Input: part model. Units: mm. Frame: model coordinates. Face numbers are marked on the shaded views. A direction names the side the tool comes from. Give positions to 0.01 mm unless a question says otherwise; leave off trailing zeros. Loops run counter-clockwise (first coordinate to the right, second up) from the corner with the lowest first, then second, coordinate; pieces in that order, holes last. Notation, with made-up numbers: (-31, -0.5) -> (11, -0.5) arc R21 cw to (11, 16.5) -> close; hole circle Ø9 at (-21.75, -36). An arc over 180 degrees is marked (long way). Answer as a JSON object with one key per item and string values.
```python
from build123d import *

# Parameters (mm, degrees)
SKETCH1_W   = 19.939
SKETCH1_H   = 40.2844
BODY_DEPTH  = 39.7002
SKETCH2_R   = 2.921
AXLE_DEPTH  = 5.6896
WINGS_START = 28.448
SKETCH3_W   = 19.939
SKETCH3_H   = 7.112
SKETCH3_R   = 2.159
WINGS_DEPTH = 3


with BuildPart() as part:
    # Sketch1 → Body (new body)
    with BuildSketch(Plane(origin=(0, 0, 0), x_dir=(1, 0, 0), z_dir=(0, 1, 0))):
        with Locations((0, -10.1422)):
            Rectangle(SKETCH1_W, SKETCH1_H)
    extrude(amount=BODY_DEPTH)

    # Sketch2 → Axle (add)
    with BuildSketch(Plane(origin=(0, 39.7002, 0), x_dir=(1, 0, 0), z_dir=(0, 1, 0))):
        Circle(SKETCH2_R)
    extrude(amount=AXLE_DEPTH)

    # Sketch3 → Wings (add)
    with BuildSketch(Plane(origin=(0, 0, 0), x_dir=(1, 0, 0), z_dir=(0, 1, 0)).offset(WINGS_START)):
        with Locations((0, 13.556)):
            Rectangle(SKETCH3_W, SKETCH3_H)
        with Locations((4.98475, 14.2672)):
            Circle(SKETCH3_R, mode=Mode.SUBTRACT)
        with Locations((-4.98475, 14.2672)):
            Circle(SKETCH3_R, mode=Mode.SUBTRACT)
    wings = extrude(amount=WINGS_DEPTH)

    # Mirror1: Wings across plane
    add(wings.mirror(Plane.XY.offset(10.1422)))


solid = part.part
```
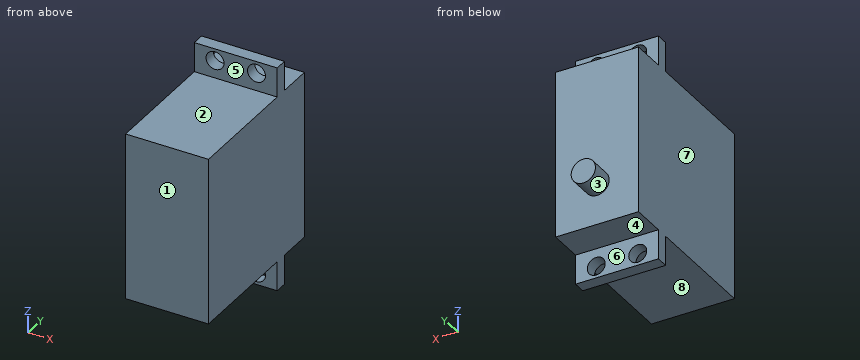
Q1. Section A-A, the plane x = 0. Return the cut outline in (y, z).
Evaluation:
{"outline": "(0, -10) -> (28.45, -10) -> (28.45, -17.11) -> (31.45, -17.11) -> (31.45, -10) -> (39.7, -10) -> (39.7, -2.92) -> (45.39, -2.92) -> (45.39, 2.92) -> (39.7, 2.92) -> (39.7, 30.28) -> (31.45, 30.28) -> (31.45, 37.4) -> (28.45, 37.4) -> (28.45, 30.28) -> (0, 30.28) -> close"}
Q2. Access query for the marked faces 5, 6, 7 and 8. Directions: +Z, -Z, +X, -X, +Y, -Y. A direction counts if a zero-diameter tool reaches every point of the face in a straight line with its end or side. Return the directions, or none.
Evaluation:
{"face 5": "+Z, +X, -X, -Y", "face 6": "-Z, +X, -X, +Y", "face 7": "+Z, -Z, -X, +Y, -Y", "face 8": "-Z, +X, -X, -Y"}
Q3. Ray query, line 1 along Y through (x, z) = (7.25, 14); line 2 along Z through (x, y) = (4, 26); line 3 along Y through (x, z) = (6.25, 32). Return the intervals inside material, ascending.
Evaluation:
{"line 1": "y = 0 to 39.7", "line 2": "z = -10 to 30.28", "line 3": "y = 28.45 to 31.45"}
Q4. Section C-C, the plane x = -5.5. Return the cut outline in (y, z), then the cut area to 3 significant figures.
Evaluation:
{"outline": "(0, -10) -> (28.45, -10) -> (28.45, -12.17) -> (31.45, -12.17) -> (31.45, -10) -> (39.7, -10) -> (39.7, 30.28) -> (31.45, 30.28) -> (31.45, 32.45) -> (28.45, 32.45) -> (28.45, 30.28) -> (0, 30.28) -> close; (28.45, -17.11) -> (31.45, -17.11) -> (31.45, -16.36) -> (28.45, -16.36) -> close; (28.45, 36.65) -> (31.45, 36.65) -> (31.45, 37.4) -> (28.45, 37.4) -> close", "area": "1,620 mm2"}
Q5. Draft query along Z for the marked faces 1, 2, 3 and 4. Return one class per face: +Z half, -Z half, draft (parallel to the pull), parting line (faces both ways), or undercut.
Evaluation:
{"face 1": "draft", "face 2": "+Z half", "face 3": "parting line", "face 4": "-Z half"}
Q6. Pin query (flat end, axial travel): pin 1 (5 mm diameter, centred on x = -4.98, z = -14.27, fed in from +Y); pin 2 (8 mm diameter, centred on x = 4.5, z = 34.5, fed in from -Y); pin 3 (10 mm diameter, centred on x = -2, y = 13.5, fed in from -Z); pin 4 (1 mm diameter, centred on y = 38.5, z = 31.5, fed in from -X). Return the tip coordinate at first contact, or that it passes through.
Evaluation:
{"pin 1": "stops at y = 31.45", "pin 2": "stops at y = 28.45", "pin 3": "stops at z = -10", "pin 4": "passes through"}
Q7. Section B-B, the plane z = 0. Return the cut outline in (x, y).
Evaluation:
{"outline": "(-9.97, 0) -> (9.97, 0) -> (9.97, 39.7) -> (2.92, 39.7) -> (2.92, 45.39) -> (-2.92, 45.39) -> (-2.92, 39.7) -> (-9.97, 39.7) -> close"}
Q8. Section D-D, the plane y = 14. Return the cut outline in (x, z), then the cut area to 3 significant figures.
Evaluation:
{"outline": "(-9.97, -10) -> (9.97, -10) -> (9.97, 30.28) -> (-9.97, 30.28) -> close", "area": "803 mm2"}
